Can you work these out from the drawing? Everything is in mm from the part's minimum corner. A direction names the side the tool comes from. Round coordinates to 2 decimals unless told otherwise and drop trailing zeros. Write each loop counter-clockwise with the first axis right and the second up, starting at its lowest first coordinate (ties: lowest second). Pieces come first, ordered by that corner, then holes.
Q1. If we section it at D-D (z = 32.5): Please give me the cut outline in (x, y).
Q2. If we section it at A-A (z = 48.15): Please give me the cut outline in (x, y).
Q3. If we section it at B-B (y = 29): Please give me the cut outline in (x, z).
Q4. I'm going to push flat-ended pins straight in: pin 1 Ø16 at (x, z) = (29.69, 28.15) entering from -Y; pin 2 Ø3 at (y, z) = (29, 23.5) entering from +X. Where does each tip first touch, or does it pass through?
Q5. For the marked faces 1 and 2, which set-ups out of +Z, -Z, +X, -X, +Y, -Y let a thin tool reach every point of the face, with its end or its side?
Q6. If we section it at C-C (x = 7): Please give me the cut outline in (y, z).
Q7. Please list where these lines run through material, in increasing order: line 1 along Y through (x, z) = (0.45, 17); line 2 along X through (y, z) = (37, 28) (1 decimal); line 3 along Y through (x, z) = (1.15, 32.5).
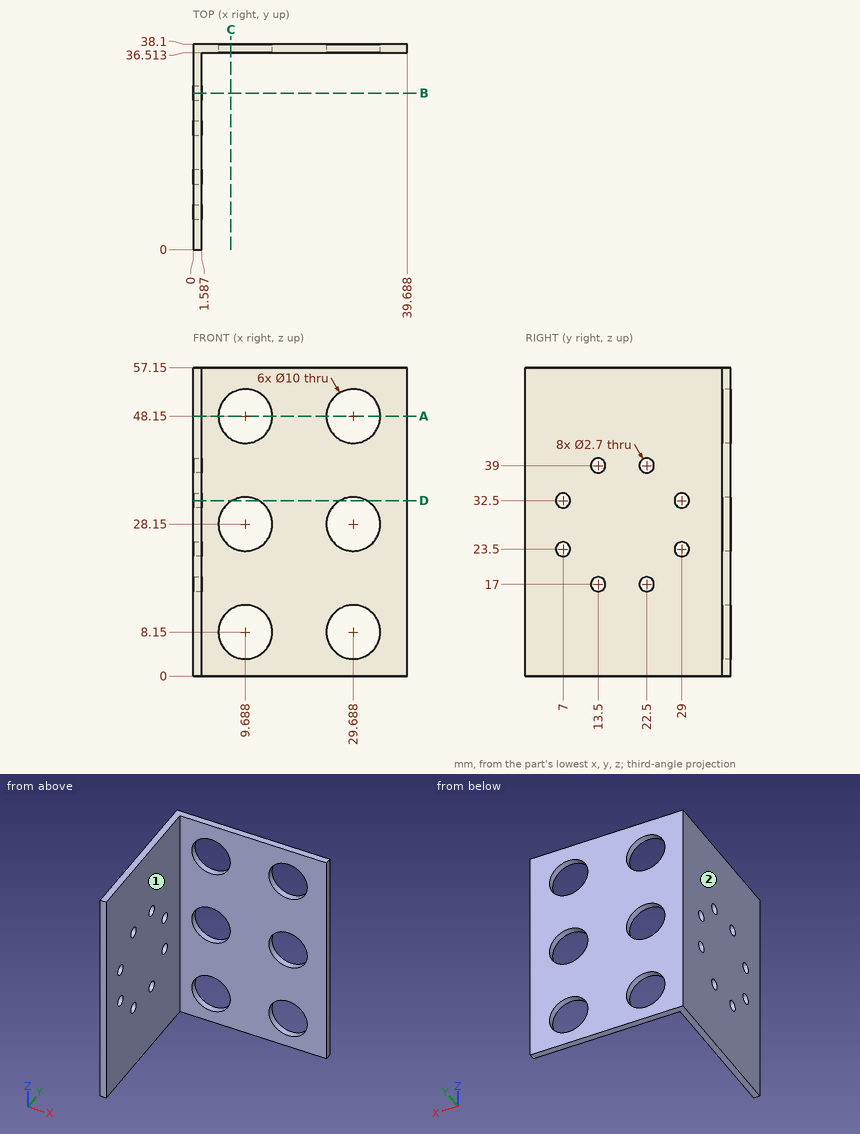
A:
1. outline: (0, 0) - (1.59, 0) - (1.59, 5.65) - (0, 5.65) - close; (0, 8.35) - (1.59, 8.35) - (1.59, 27.65) - (0, 27.65) - close; (0, 30.35) - (1.59, 30.35) - (1.59, 36.51) - (7.22, 36.51) - (7.22, 38.1) - (0, 38.1) - close; (12.15, 36.51) - (27.22, 36.51) - (27.22, 38.1) - (12.15, 38.1) - close; (32.15, 36.51) - (39.69, 36.51) - (39.69, 38.1) - (32.15, 38.1) - close
2. outline: (0, 0) - (1.59, 0) - (1.59, 36.51) - (4.69, 36.51) - (4.69, 38.1) - (0, 38.1) - close; (14.69, 36.51) - (24.69, 36.51) - (24.69, 38.1) - (14.69, 38.1) - close; (34.69, 36.51) - (39.69, 36.51) - (39.69, 38.1) - (34.69, 38.1) - close
3. outline: (0, 0) - (1.59, 0) - (1.59, 22.15) - (0, 22.15) - close; (0, 24.85) - (1.59, 24.85) - (1.59, 31.15) - (0, 31.15) - close; (0, 33.85) - (1.59, 33.85) - (1.59, 57.15) - (0, 57.15) - close
4. pin 1: stops at y = 36.51
4. pin 2: stops at x = 1.59
5. face 1: +Z, -Z, +X, -Y
5. face 2: +Z, -Z, -X, +Y, -Y
6. outline: (36.51, 0) - (38.1, 0) - (38.1, 3.93) - (36.51, 3.93) - close; (36.51, 12.37) - (38.1, 12.37) - (38.1, 23.93) - (36.51, 23.93) - close; (36.51, 32.37) - (38.1, 32.37) - (38.1, 43.93) - (36.51, 43.93) - close; (36.51, 52.37) - (38.1, 52.37) - (38.1, 57.15) - (36.51, 57.15) - close
7. line 1: y = 0 to 12.15, 14.85 to 21.15, 23.85 to 38.1
7. line 2: x = 0 to 4.7, 14.7 to 24.7, 34.7 to 39.7
7. line 3: y = 0 to 5.65, 8.35 to 27.65, 30.35 to 38.1
